Geometry check sheet. Reference: the model listing, model coordinates, mm. A direction names the side the tool comes from. Round coordinates to 2 decimals unless told otherwise and drop trailing zeros. Loops run counter-clockwise (first coordinate to the right, second up) from the corner with the lowest first, then second, coordinate; pieces in that order, holes last. Notation, with made-up numbers: (-17.75, 6.25) - (-8.75, 6.25) arc R22 ccw to (-8.75, 19.25) - close; hole circle Ø5 at (76, 89). An arc over 180 degrees is marked (long way). Answer as CSV lines item,"result". Start each with the question number.
1) Cross-section at B-B on x = 20. Record the boundary of the cut face in (y, z) (1 decimal).
2) Draft check along X on faces 3 (the flat face through (9, 0, 48)), 4 (the flat face through (30.905, 11.943, 48.215)), 5 (the cylindrical face through (38.859, 1.203, 48.215)). Enter one of: released by +X, released by -X, zero draft, split by the parting line, or undercut.
3) Depth check by flat-ended pin: P1, Ø0.7, axis at y = 38, z = 30, coming from the +X side; P2, Ø1.5, axis at y = 37.5, z = 39.5, coming from the -X side; P3, Ø6, axis at x = 21.5, z = 52, coming from the -Y side. Enter the tip coordinate at first touch or a pass-through.
4) Access from +Z, -Z, +X, -X, +Y, -Y to the whole of each face (thin tool, end or side, straight path). Record for faces 1 (the flat face through (15, 20, 97.8)), 2 (the flat face through (12, 35.68, 48)).
5) Cross-section at A-A on y = 20. Record the boundary of the cut face in (x, z) (3 decimals).
6) Thickness scan on line 1 along Y through (x, z) = (20, 43) (1 decimal); line 2 along Y through (x, z) = (15.5, 68.5); line 3 along X through (y, z) = (30.5, 63.5). Record the ranges inside material, lowest first.
Autodesk Fusion 360 part; units mm, degrees
sketch "Sketch1" plane through (0, 0, 0) normal (0, 0, 1) x (1, 0, 0)
  line L0 (4, 0) -> (14.435, 0)
  line L1 (40, 0) -> (40, 36)
  line L2 (36, 40) -> (0, 40)
  line L3 (0, 40) -> (0, 4)
  line L4 (0, 0) -> (0, 20)
  line L5 (0, 40) -> (20, 40)
  circle A0 centre (20, 20) radius 3.405
  line L6 (40, 40) -> (24.065, 40)
  line L7 (40, 40) -> (25.565, 40)
  line L8 (40, 40) -> (40, 25.565)
  line L9 (38.5, 24.065) -> (37.18, 24.065)
  line L10 (24.065, 38.5) -> (24.065, 37.18)
  line L11 (25.565, 35.68) -> (30.4344, 35.68)
  line L12 (35.68, 25.565) -> (35.68, 30.2904)
  line L13 (20, 20) -> (20, 40)
  line L14 (20, 20) -> (0, 20)
  line L15 (20, 20) -> (20, 0)
  line L16 (20, 20) -> (40, 20)
  line L17 (14.435, 35.68) -> (9.5498, 35.68)
  line L18 (15.935, 38.5) -> (15.935, 37.18)
  line L19 (4, 40) -> (14.435, 40)
  line L20 (0, 36) -> (0, 25.565)
  line L21 (1.5, 24.065) -> (2.8205, 24.065)
  line L22 (4.3205, 25.5645) -> (4.3219, 30.271)
  line L23 (25.565, 4.32) -> (1890698.4728, 3)
  line L24 (24.065, 1.5) -> (24.065, 2.82)
  line L25 (36, 0) -> (25.565, 0)
  line L26 (40, 4) -> (40, 14.435)
  line L27 (38.5, 15.935) -> (37.18, 15.935)
  line L28 (35.68, 14.435) -> (35.68, 9.7153)
  line L29 (14.435, 4.32) -> (9.7085, 4.32)
  line L30 (15.935, 1.5) -> (15.935, 2.82)
  line L31 (0, 0) -> (15.935, 0)
  line L32 (1.5, 15.935) -> (2.82, 15.935)
  line L33 (4.32, 14.435) -> (4.32, 9.5656)
  line L34 (0, 14.435) -> (0, 0)
  line L35 (0, 0) -> (15.935, 0)
  line L36 (5.9379, 30.9139) -> (12.3015, 24.1858)
  line L37 (8.8698, 34.1008) -> (15.0285, 27.5893)
  line L38 (30.9385, 5.9323) -> (24.4402, 12.1491)
  line L39 (33.9887, 8.9927) -> (27.7337, 14.9768)
  line L40 (5.903, 8.8892) -> (12.2663, 14.9767)
  line L41 (9.0615, 5.9323) -> (15.5598, 12.1491)
  line L42 (31.1111, 34.0973) -> (24.8873, 27.5855)
  line L43 (33.957, 30.8226) -> (27.7021, 24.2782)
  line L44 (27.425, 23.5872) -> (27.425, 15.6993)
  line L45 (16.2511, 12.4265) -> (23.7489, 12.4265)
  line L46 (12.575, 15.6993) -> (12.575, 23.4986)
  line L47 (15.7551, 27.2765) -> (24.1644, 27.2765)
  line L48 (35.68, 30.1316) -> (35.68, 30.2853)
  line L49 (34.0667, 30.9373) -> (34.0632, 30.9337)
  arc A1 (33.9887, 8.9927) -> (35.68, 9.7153) centre (34.68, 9.7153) ccw
  line L50 (35.68, 7.3747) -> (35.68, 9.7153)
  arc A2 (27.7021, 24.2782) -> (27.425, 23.5872) centre (28.425, 23.5872) ccw
  arc A3 (35.68, 30.2904) -> (34.0667, 30.9373) centre (34.7436, 30.2904) ccw
  arc A4 (5.9379, 30.9139) -> (4.3219, 30.271) centre (5.2579, 30.2707) ccw
  arc A5 (12.575, 23.4986) -> (12.3015, 24.1858) centre (11.575, 23.4986) ccw
  arc A6 (12.2663, 14.9767) -> (12.575, 15.6993) centre (11.575, 15.6993) ccw
  arc A7 (4.32, 9.5656) -> (5.903, 8.8892) centre (5.256, 9.5656) ccw
  arc A8 (9.0615, 5.9323) -> (9.7085, 4.32) centre (9.7085, 5.256) ccw
  arc A9 (30.2914, 4.32) -> (30.9385, 5.9323) centre (30.2914, 5.256) ccw
  arc A10 (24.4402, 12.1491) -> (23.7489, 12.4265) centre (23.7489, 11.4265) ccw
  arc A11 (16.2511, 12.4265) -> (15.5598, 12.1491) centre (16.2511, 11.4265) ccw
  arc A12 (27.425, 15.6993) -> (27.7337, 14.9768) centre (28.425, 15.6993) ccw
  arc A13 (24.1644, 27.2765) -> (24.8873, 27.5855) centre (24.1644, 28.2765) ccw
  arc A14 (15.0285, 27.5893) -> (15.7551, 27.2765) centre (15.7551, 28.2765) ccw
  arc A15 (37.18, 15.935) -> (35.68, 14.435) centre (37.18, 14.435) ccw
  arc A16 (40, 14.435) -> (38.5, 15.935) centre (38.5, 14.435) ccw
  arc A17 (35.68, 25.565) -> (37.18, 24.065) centre (37.18, 25.565) ccw
  arc A18 (38.5, 24.065) -> (40, 25.565) centre (38.5, 25.565) ccw
  arc A19 (25.565, 40) -> (24.065, 38.5) centre (25.565, 38.5) ccw
  arc A20 (24.065, 37.18) -> (25.565, 35.68) centre (25.565, 37.18) ccw
  arc A21 (14.435, 35.68) -> (15.935, 37.18) centre (14.435, 37.18) ccw
  arc A22 (15.935, 38.5) -> (14.435, 40) centre (14.435, 38.5) ccw
  arc A23 (2.8205, 24.065) -> (4.3205, 25.5645) centre (2.8205, 25.565) ccw
  arc A24 (0, 25.565) -> (1.5, 24.065) centre (1.5, 25.565) ccw
  arc A25 (4.32, 14.435) -> (2.82, 15.935) centre (2.82, 14.435) ccw
  arc A26 (1.5, 15.935) -> (0, 14.435) centre (1.5, 14.435) ccw
  arc A27 (15.935, 2.82) -> (14.435, 4.32) centre (14.435, 2.82) ccw
  arc A28 (1890698.4728, 0) -> (1890698.4728, 3) centre (1890698.4728, 1.5) ccw
  arc A29 (24.065, 1.5) -> (25.565, 0) centre (25.565, 1.5) ccw
  arc A30 (14.435, 0) -> (15.935, 1.5) centre (14.435, 1.5) ccw
  arc A31 (25.565, 4.32) -> (24.065, 2.82) centre (25.565, 2.82) ccw
  arc A32 (4, 40) -> (0, 36) centre (4, 36) ccw
  arc A33 (0, 4) -> (4, 0) centre (4, 4) ccw
  arc A34 (36, 0) -> (40, 4) centre (36, 4) ccw
  arc A35 (40, 36) -> (36, 40) centre (36, 36) ccw
  arc A36 (9.5498, 35.68) -> (8.8698, 34.1008) centre (9.5498, 34.744) ccw
  arc A37 (31.1111, 34.0973) -> (30.4344, 35.68) centre (30.4344, 34.744) ccw
  line L51 (40, 25.1972) -> (40, 36)
  line L52 (33.957, 30.8226) -> (34.0632, 30.9337)
  point P0 (20, 20)
  point P1 (40, 24.065)
  point P2 (35.68, 24.065)
  point P3 (24.065, 35.68)
  point P4 (35.68, 32.6253)
  point P5 (35.68, 7.3747)
  dimension "d1" = 40
  dimension "d2" = 40
  dimension "d8" = 15.935
  dimension "d9" = 15.935
  dimension "d10" = 4.32
  dimension "d11" = 4.32
  dimension "d16" = 90
  dimension "d17" = 90
  dimension "d22" = 4.32
  dimension "d23" = 4.32
  dimension "d24" = 4.32
  dimension "d25" = 4.32
  dimension "d26" = 8.13
  dimension "d27" = 4.32
  dimension "d28" = 14.85
  dimension "d29" = 14.85
  dimension "d30" = 7.425
  dimension "d31" = 25.2506
  dimension "d32" = 2.34
  dimension "d33" = 2.34
  dimension "d35" = 1
  dimension "d36" = 20.57
  dimension "d37" = 1
  dimension "d38" = 7.9779
  dimension "d39" = 0.9364
  dimension "d40" = 0.936
  dimension "d41" = 1
  dimension "d42" = 1
  dimension "d43" = 0.936
  dimension "d44" = 0.936
  dimension "d45" = 0.936
  dimension "d46" = 1
  dimension "d47" = 1
  dimension "d48" = 1
  dimension "d49" = 1
  dimension "d50" = 1
  dimension "d51" = 1.5
  dimension "d52" = 1.5
  dimension "d53" = 1.5
  dimension "d54" = 1.5
  dimension "d55" = 1.5
  dimension "d56" = 1.5
  dimension "d57" = 1.5
  dimension "d58" = 1.5
  dimension "d59" = 4
  dimension "d60" = 4
  dimension "d61" = 0.936
  dimension "d62" = 0.936
extrude "Extrude1" add sketch "Sketch1" along normal blind 97.8 contours L0 L3 L4 A0 L14 L15 L29 L30 L31 L32 L33 L34 L35 L40 L41 L45 L46 A6 A7 A8 A11 A25 A26 A27 A30 A33 | L2 L3 L5 A0 L13 L14 L17 L18 L19 L20 L21 L22 L36 L37 L46 L47 A4 A5 A14 A21 A22 A23 A24 A32 A36 | L1 L2 A0 L6 L7 L8 L9 L10 L11 L12 L13 L16 L42 L43 L44 L47 L48 L49 A2 A3 A13 A17 A18 A19 A20 A35 A37 L51 L52 | L1 A0 L15 L16 L23 L26 L27 L28 L38 L39 L44 L45 A1 A9 A10 A12 A15 A16 | L1 L23 L24 L25 L26 A29 A31 A34
Answer block:
1,outline,"(12.4, 0) - (16.6, 0) - (16.6, 97.8) - (12.4, 97.8) - close; (23.4, 0) - (27.3, 0) - (27.3, 97.8) - (23.4, 97.8) - close"
2,face 3,"zero draft"
2,face 4,"undercut"
2,face 5,"released by +X"
3,P1,"stops at x = 39.64"
3,P2,"stops at x = 0.07"
3,P3,"stops at y = 0.44"
4,face 1,"+Z, +X, -X, +Y, -Y"
4,face 2,"+Z, -Z"
5,outline,"(12.575, 0) - (16.595, 0) - (16.595, 97.8) - (12.575, 97.8) - close; (23.405, 0) - (27.425, 0) - (27.425, 97.8) - (23.405, 97.8) - close"
6,line 1,"y = 12.4 to 16.6, 23.4 to 27.3"
6,line 2,"y = 0.44 to 3.88, 12.09 to 27.31, 36.12 to 39.56"
6,line 3,"x = 0 to 4.35, 6.33 to 12.28, 27.67 to 33.65, 35.66 to 40"
